from build123d import *

# Parameters (mm, degrees)
SKETCH1_W           = 76.2
SKETCH1_H           = 63.5
BOSS_EXTRUDE1_DEPTH = 6.35
SKETCH2_R           = 3.175
CUT_EXTRUDE1_DEPTH  = 50.99995
BOSS_EXTRUDE2_DEPTH = 63.5
SKETCH4_W           = 63.5
SKETCH4_H           = 6.35
BOSS_EXTRUDE3_DEPTH = 76.2


with BuildPart() as part:
    # Sketch1 → Boss-Extrude1 (new body)
    with BuildSketch(Plane(origin=(0, 0, 0), x_dir=(1, 0, 0), z_dir=(0, 1, 0))):
        Rectangle(SKETCH1_W, SKETCH1_H)
    extrude(amount=BOSS_EXTRUDE1_DEPTH)

    # Sketch2 → Cut-Extrude1 (cut, through all)
    with BuildSketch(Plane(origin=(0, 6.35, 0), x_dir=(1, 0, 0), z_dir=(0, 1, 0))):
        with Locations(Location((0, 0, 0), (0, 0, 270))):
            Circle(SKETCH2_R)
    extrude(amount=-CUT_EXTRUDE1_DEPTH, mode=Mode.SUBTRACT)

    # Sketch3 → Boss-Extrude2 (add)
    with BuildSketch(Plane.XY.offset(31.75)):
        Polygon((38.1, 6.35), (190.5, 304.8), (190.5, 298.45), (38.1, 0), align=None)
    extrude(amount=-BOSS_EXTRUDE2_DEPTH)

    # Sketch4 → Boss-Extrude3 (add)
    with BuildSketch(Plane(origin=(190.5, 0, 0), x_dir=(0, 0, -1), z_dir=(1, 0, 0))):
        with Locations((0, 301.625)):
            Rectangle(SKETCH4_W, SKETCH4_H)
    extrude(amount=BOSS_EXTRUDE3_DEPTH)


solid = part.part
Verification items for the finished model (mm, model axes). A direction names the side the tool comes from. Round coordinates to 2 decimals unless told otherwise and drop trailing zeros. Write each loop counter-clockwise with the first axis right and the second up, starting at its lowest first coordinate (ties: lowest second). Pieces come first, ordered by that corner, then holes.
(1) Depth check by flat-ended pin: pin 1 Ø10 at (x, z) = (43, 5) entering from +Y; pin 2 Ø4 at (x, z) = (108.5, -12.5) entering from -Y; pin 3 Ø2 at (x, z) = (31.5, 14) entering from +Y. Enter the tip coordinate at first touch or a pass-through.
Returned:
pin 1: stops at y = 25.74
pin 2: stops at y = 133.95
pin 3: stops at y = 6.35
(2) Section check A-A (z = 15.5). Enter the section's corners in (x, y), plus the area to 3 significant figures.
Returned:
outline: (-38.1, 0) - (38.1, 0) - (190.5, 298.45) - (266.7, 298.45) - (266.7, 304.8) - (190.5, 304.8) - (38.1, 6.35) - (-38.1, 6.35) - close
area: 1,940 mm2
(3) Material ranges on line 1 (Y direction, x = 245, z = 28); line 2 (X direction, y = 3, z = 0) (3 decimals); line 3 (X direction, y = 4, z = 0) (3 decimals), recorded low to high.
Returned:
line 1: y = 298.45 to 304.8
line 2: x = -38.1 to -3.175, 3.175 to 39.632
line 3: x = -38.1 to -3.175, 3.175 to 40.143
(4) Section check C-C (y = 261). Enter the section's corners in (x, z), plus the area to 3 significant figures.
Returned:
outline: (168.13, -31.75) - (171.38, -31.75) - (171.38, 31.75) - (168.13, 31.75) - close
area: 206 mm2
(5) Access from +Z, -Z, +X, -X, +Y, -Y to the whole of each face (thin tool, end or side, straight path). Record for faces 1 (the flat face through (228, 298.45, 0)), 2 (the flat face through (-1, 6.35, -8)), 3 (the flat face through (80, 84, -31.75)).
Returned:
face 1: +Z, -Z, +X, -Y
face 2: +Z, -Z, -X, +Y
face 3: -Z, +X, -X, +Y, -Y
(6) Section check B-B (x = 105.5). Enter the section's corners in (y, z), plus the area to 3 significant figures.
Returned:
outline: (131.99, -31.75) - (138.34, -31.75) - (138.34, 31.75) - (131.99, 31.75) - close
area: 403 mm2
